from build123d import *

# Parameters (mm, degrees)
SKETCH1_W           = 25.4
SKETCH1_H           = 25.4
BOSS_EXTRUDE1_DEPTH = 6.35
SKETCH2_W           = 6.4
SKETCH2_H           = 3.2
BOSS_EXTRUDE2_DEPTH = 10
SKETCH3_R           = 2.498733
CUT_EXTRUDE1_DEPTH  = 20.1


with BuildPart() as part:
    # Sketch1 → Boss-Extrude1 (new body)
    with BuildSketch(Plane.XY):
        Rectangle(SKETCH1_W, SKETCH1_H)
    extrude(amount=BOSS_EXTRUDE1_DEPTH)

    # Sketch2 → Boss-Extrude2 (add)
    with BuildSketch(Plane(origin=(0, 0, 0), x_dir=(-1, 0, 0), z_dir=(0, 0, -1))):
        with Locations((0, 4.8)):
            Rectangle(SKETCH2_W, SKETCH2_H)
        with Locations((0, -4.8)):
            Rectangle(SKETCH2_W, SKETCH2_H)
    extrude(amount=BOSS_EXTRUDE2_DEPTH)

    # Sketch3 → Cut-Extrude1 (cut, through all)
    with BuildSketch(Plane(origin=(0, 6.4, 0), x_dir=(1, 0, 0), z_dir=(0, 1, 0))):
        with Locations((0, 6.830385607)):
            Circle(SKETCH3_R)
    extrude(amount=-CUT_EXTRUDE1_DEPTH, mode=Mode.SUBTRACT)


solid = part.part
Input: part model. Units: mm. Frame: model coordinates. A direction names the side the tool comes from. Coordinates: 2 decimals unless noted, no trailing zeros. Order: outer loops, then holes, each group sorted by start corner. A loop starts at its lowest first (then second) coordinate and runs counter-clockwise, first axis right, second up. Notation, with made-up numbers: M 2,64.5 L 48,64.5 A24 cw 48,86.5 Z; hole C -20.5,33.5 d10. An arc over 180 degrees is marked long. One line per question, with ' | ' between items.
Item 1: Draft query along Y for faces 6 (the flat face through (12.7, 0, 3)), 7 (the flat face through (0, -12.7, 3)), 8 (the flat face through (0, -3.2, -4)). Return one class per face: released by +Y, released by -Y, zero draft, split by the parting line, or undercut.
Geometry results:
face 6: zero draft | face 7: released by -Y | face 8: undercut
Item 2: Section C-C (y = 1). Output: boundary loops of the cut face in (x, z).
Geometry results:
outline: M -12.7,0 L 12.7,0 L 12.7,6.35 L -12.7,6.35 Z
Item 3: Section A-A (x = 0). Output: boundary loops of the cut face in (y, z).
Geometry results:
outline: M -12.7,0 L -6.4,0 L -6.4,-4.33 L -3.2,-4.33 L -3.2,0 L 3.2,0 L 3.2,-4.33 L 6.4,-4.33 L 6.4,0 L 12.7,0 L 12.7,6.35 L -12.7,6.35 Z; M -6.4,-10 L -3.2,-10 L -3.2,-9.33 L -6.4,-9.33 Z; M 3.2,-10 L 6.4,-10 L 6.4,-9.33 L 3.2,-9.33 Z
Item 4: Section B-B (z = -3.5). Output: boundary loops of the cut face in (x, y).
Geometry results:
outline: M -3.2,-6.4 L 3.2,-6.4 L 3.2,-3.2 L -3.2,-3.2 Z; M -3.2,3.2 L 3.2,3.2 L 3.2,6.4 L -3.2,6.4 Z
Item 5: Pin query (flat end, axial travel): pin 1 (1.5 mm diameter, centred on y = -6.5, z = -3, fed in from +X); pin 2 (3 mm diameter, centred on x = 0.5, z = -3.5, fed in from -Y); pin 3 (3 mm diameter, centred on x = 1.5, z = -4.5, fed in from +Y); pin 4 (4 mm diameter, centred on x = 0, z = -6.83, fed in from +Y). Return the tip coordinate at first contact, or that it passes through.
Geometry results:
pin 1: stops at x = 3.2 | pin 2: stops at y = -6.4 | pin 3: stops at y = 6.4 | pin 4: passes through
Item 6: Reachability of faces 1 (the flat face through (3.2, -5, -5)), 2 (the flat face through (-3.2, -5, -5)), 3 (the flat face through (0, 6.4, -4)), 4 (the flat face through (0, -6.4, -4)), 5 (the flat face through (0, 3.2, -4)) from +Z, -Z, +X, -X, +Y, -Y: full face, straight path, thin tool, end or side. Return the list, or none.
Geometry results:
face 1: -Z, +X, +Y, -Y | face 2: -Z, -X, +Y, -Y | face 3: -Z, +X, -X, +Y | face 4: -Z, +X, -X, -Y | face 5: -Z, +X, -X
Item 7: Ray query, line 1 along Z through (x, y) = (0, 4.1); line 2 along Y through (x, z) = (-0.75, -4); line 3 along Z through (x, y) = (-5.25, 0.25). Return the intervals inside material, ascending.
Geometry results:
line 1: z = -10 to -9.33, -4.33 to 6.35 | line 2: y = -6.4 to -3.2, 3.2 to 6.4 | line 3: z = 0 to 6.35
